Model file for the job. Use its own axes, mm. Face numbers are marked on the shaded views. A direction names the side the tool comes from. Round coordinates to 2 decimals unless told otherwise and drop trailing zeros. Loops run counter-clockwise (first coordinate to the right, second up) from the corner with the lowest first, then second, coordinate; pieces in that order, holes last. Notation, with made-up numbers: M 87,5.25 L 131,5.25 A33 ccw 131,36.25 Z; hole C 57,63 d11. An arc over 180 degrees is marked long. Answer in a Markdown table with one row per item.
Autodesk Inventor part; units mm, degrees
ref_plane "YZ Plane" through (0, 0, 0) normal (1, 0, 0) x (0, 1, 0)
ref_plane "XZ Plane" through (0, 0, 0) normal (0, 1, 0) x (-1, 0, 0)
ref_plane "XY Plane" through (0, 0, 0) normal (0, 0, 1) x (1, 0, 0)
sketch "Sketch1" plane through (0, 0, 0) normal (0, 1, 0) x (-1, 0, 0)
  circle A0 centre (0, 0) radius 14.75
  line L0 (0, -14.75) -> (0, -12.9)
  circle A1 centre (0, 0) radius 12.9
  dimension "d0" = 29.5
  dimension "d1" = 1.85
extrude "Extrusion1" add sketch "Sketch1" along normal blind 1.2 contours A1 | A0
sketch "Sketch2" plane through (0, 1.2, 0) normal (0, 1, 0) x (1, 0, 0)
  circle A0 centre (0, 0) radius 14.75
  line L0 (0, 14.75) -> (0, 12.9)
  circle A1 centre (0, 0) radius 12.9
  dimension "d4" = 1.85
extrude "Extrusion2" add sketch "Sketch2" along normal blind 11.25
fillet "Fillet1" radius 1.2 1 edges at (14.75, 0, 0)
properties part number "Bottle"
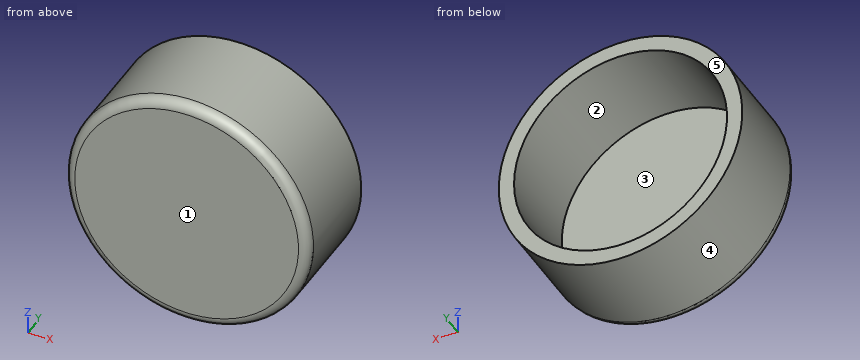
1. Saw through at A-A (y = 5). Write the cut outline in (x, z), and give its area (3 significant figures).
Verdict:
| item | result |
|---|---|
| outline | C 0,0 d29.5; hole C 0,0 d25.8 |
| area | 161 mm² |
2. Wall check: probe 1 along Z at (x, y) = (0, 7.5); probe 2 along Z at (x, y) = (9.25, 7); probe 3 along X at (y, z) = (7.5, -7.25). Give the ranges that are in metal, low to high.
Verdict:
| item | result |
|---|---|
| probe 1 | z = -14.75 to -12.9, 12.9 to 14.75 |
| probe 2 | z = -11.49 to -8.99, 8.99 to 11.49 |
| probe 3 | x = -12.85 to -10.67, 10.67 to 12.85 |
3. Mould opens along Z. For the marked faces 3, 4 and 5 say: +Z half, -Z half, draft (parallel to the pull), parting line (faces both ways), or undercut.
Verdict:
| item | result |
|---|---|
| face 3 | undercut |
| face 4 | parting line |
| face 5 | draft |
4. Tool access for the marked faces 1 and 2: list every direction of +Z, -Z, +X, -X, +Y, -Y with a clear straight run to the whole face (end or side of a thin tool).
Verdict:
| item | result |
|---|---|
| face 1 | +Z, -Z, +X, -X, -Y |
| face 2 | +Y |
5. Pin check, flat tips, straight feed: pin 1 (10 mm diameter, centred on x = -4.5, z = 3.5, fed in from +Y); pin 2 (2 mm diameter, centred on y = 3, z = 3.5, fed in from +X); pin 3 (5 mm diameter, centred on y = 2, z = 4, fed in from +X). Stop position of each tip, or through.
Verdict:
| item | result |
|---|---|
| pin 1 | stops at y = 1.2 |
| pin 2 | stops at x = 14.54 |
| pin 3 | stops at x = 14.67 |
